For this review, take the finished solid that the model builds, in its own axes (mm). A direction names the side the tool comes from. Round coordinates to 2 decimals unless told otherwise and drop trailing zeros. Loops run counter-clockwise (first coordinate to the right, second up) from the corner with the lowest first, then second, coordinate; pieces in that order, holes last. Notation, with made-up numbers: (-14, -24) -> (22, -24) arc R32 ccw to (22, 5) -> close; hole circle Ø2 at (0, 64.5). An arc over 180 degrees is marked (long way). Use one line per item in the form item = value. Start each with the question number.
from build123d import *

# Parameters (mm, degrees)
F1_DEPTH = 483.87
F2_R     = 127
F3_R     = 38.1
F4_DEPTH = 99.06
F5_R     = 63.5
F6_DEPTH = 360.68


with BuildPart() as f1:
    # F0 (on Front) → F1 (new body)
    with BuildSketch(Plane.XZ):
        with BuildLine():
            Line((514.1757349964, 629.7824745688), (112.5849840774, 137.8984752597))
            ThreePointArc((112.5849840774, 137.8984752597), (101.7025756268, 48.26), (178.0206957594, 0))
            Line((178.0206957594, 0), (1448.0206957594, 0))
            Line((1448.0206957594, 0), (1448.0206957594, 36.4776443297))
            Line((1448.0206957594, 36.4776443297), (178.0206957594, 36.4776443297))
            ThreePointArc((178.0206957594, 36.4776443297), (134.6581275023, 63.8980988751), (140.8413141219, 114.8290507272))
            Line((140.8413141219, 114.8290507272), (542.4320650409, 606.7130500363))
            Line((542.4320650409, 606.7130500363), (514.1757349964, 629.7824745688))
        make_face()
    extrude(amount=F1_DEPTH)

    # F2
    f2_edges = [f1.edges().sort_by_distance(p)[0] for p in [
        (1448.020696, -483.87, 18.238822),
        (1448.020696, 0, 18.238822),
        (528.3039, -483.87, 618.247762),
        (528.3039, 0, 618.247762),
    ]]
    fillet(f2_edges, radius=F2_R)

    # F3 (on face) → F4 (cut)
    with BuildSketch(Plane(origin=(0, 0, 0), x_dir=(0, -1, 0), z_dir=(-0.7746204714, 0, 0.6324263794))):
        with Locations((114.3, 622.5206957594)):
            Circle(F3_R)
        with Locations((369.57, 622.5206957594)):
            Circle(F3_R)
    extrude(amount=-F4_DEPTH, mode=Mode.SUBTRACT)

    # F5 (on face) → F6 (cut)
    with BuildSketch(Plane.XY.offset(36.4776443297)):
        with Locations((635.2206957594, -241.935)):
            Circle(F5_R)
        with BuildLine():
            ThreePointArc((1270.2206957594, -305.435), (1333.7206957594, -241.935), (1270.2206957594, -178.435))
            Line((1270.2206957594, -178.435), (1016.2206957594, -178.435))
            ThreePointArc((1016.2206957594, -178.435), (952.7206957594, -241.935), (1016.2206957594, -305.435))
            Line((1016.2206957594, -305.435), (1270.2206957594, -305.435))
        make_face()
    extrude(amount=-F6_DEPTH, mode=Mode.SUBTRACT)


solid = f1.part
Item 1: Take a section at A-A on x = 1235. Give the boundary of the cut face in (y, z) (3 decimals).
Item 2: Take a section at C-C on x = 888. Give the boundary of the cut face in (y, z).
Item 3: Take a section at D-D on z = 401. Give the boundary of the cut face in (x, y).
Item 4: Take a section at B-B on y = -106.5. Give the boundary of the cut face in (x, z).
Item 5: Draft analysis for pull direction Y (two halves, no side actions). For faces 1 (the cylindrical face through (1411.805, -445.68, 18.494)), 2 (the flat face through (822, -239, 36.478)), 3 (the flat face through (1145, -178.435, 18)), 4 (the flat face through (1141, -305.435, 18)), state which applies: +Y half, -Y half, draft (parallel to the pull), parting line (faces both ways), or undercut.
Item 6: Machinability: for faces 5 (the flat face through (568, -483.87, 31)), 6 (the cylindrical face through (952.736, -240.539, 18.494)), 7 (the flat face through (338.826, -238.548, 357.328)), which of the approach directions +Z, -Z, +X, -X, +Y, -Y give a long, thin tool a straight path to every point of the face, cutting with its end or side? Answer none if there is none.
Item 7: Wall thickness on line 1 (Z direction, x = 1345.5, y = -117); line 2 (Z direction, x = 273, y = -143); line 3 (Z direction, x = 490, y = -344.5): over which ranges is each line inside the solid? List them lowest first.
Item 8: For P1, Ø5, axis at x = 902.5, y = -184.5, coming from the +Z side; P2, Ø6, axis at y = -348, z = 243.5, coming from the +X side; P3, Ø12, axis at y = -342, z = 216, coming from the +X side, all flat-tipped, find the tip position at first contact; note any pin that passes through.
Results:
q1.outline = (-483.87, 0) -> (-305.435, 0) -> (-305.435, 36.478) -> (-483.87, 36.478) -> close; (-178.435, 0) -> (0, 0) -> (0, 36.478) -> (-178.435, 36.478) -> close
q2.outline = (-483.87, 0) -> (0, 0) -> (0, 36.48) -> (-483.87, 36.48) -> close
q3.outline = (327.39, -483.87) -> (374.48, -483.87) -> (374.48, 0) -> (327.39, 0) -> close
q4.outline = (112.58, 137.9) arc R84.47 ccw to (178.02, 0) -> (1446.36, 0) -> (1446.36, 36.48) -> (178.02, 36.48) arc R48 cw to (140.84, 114.83) -> (398.37, 430.26) -> (370.11, 453.33) -> close; (417.28, 511.11) -> (445.54, 488.04) -> (541.38, 605.42) -> (513.12, 628.49) -> close
q5.face_1 = -Y half
q5.face_2 = draft
q5.face_3 = undercut
q5.face_4 = undercut
q6.face_5 = +Z, -Z, +X, -X, -Y
q6.face_6 = +Z, -Z
q6.face_7 = +X, +Y, -Y
q7.line_1 = 0 to 36.48
q7.line_2 = 0 to 36.48, 276.7 to 334.38
q7.line_3 = 0 to 36.48, 542.49 to 600.17
q8.P1 = 36.48
q8.P2 = 248.34
q8.P3 = 228.34
